Design review of the part built by this model. Coordinates are the model's own, in mm. A direction names the side the tool comes from. Coordinates: 2 decimals unless noted, no trailing zeros. Order: outer loops, then holes, each group sorted by start corner. A loop starts at its lowest first (then second) coordinate and runs counter-clockwise, first axis right, second up. Notation, with made-up numbers: M 43.5,-32 L 97.5,-32 A26 ccw 97.5,-16 Z; hole C 48.5,48.5 d2. An arc over 180 degrees is marked long. Answer as a JSON object with one key per item and string values.
from build123d import *

# Parameters (mm, degrees)
F2_W     = 2
F2_H     = 35.500896
F3_DEPTH = 89.001
F6_DEPTH = 89.001


with BuildPart() as f1:
    # F0 (on Front) → F1 (revolve)
    with BuildSketch(Plane.XZ):
        Polygon((-44.5, 45), (-44.5, 30), (44.5, 30), (44.5, 57.508134), align=None)
    revolve(axis=Axis((4.300002, 0, 0), (1, 0, 0)))

    # F2 (on face) → F3 (cut, through all)
    with BuildSketch(Plane.YZ.offset(44.5)):
        with Locations((0, -46.971067)):
            Rectangle(F2_W, F2_H)
    extrude(amount=-F3_DEPTH, mode=Mode.SUBTRACT)

    # F5 (on face) → F6 (cut, through all)
    with BuildSketch(Plane.YZ.offset(44.5)):
        Polygon((-9.3801, 23.522235), (-19.162689, 33.304824), (-33.304824, 19.162689), (-23.522235, 9.3801), align=None)
    extrude(amount=-F6_DEPTH, mode=Mode.SUBTRACT)


solid = f1.part
1) Insertion check: pin 1 Ø6 at (x, z) = (22, 20.5) entering from +Y; pin 2 Ø3 at (x, y) = (6, 46) entering from -Z; pin 3 Ø22 at (x, z) = (-1, -41) entering from -Y; pin 4 Ø10 at (y, z) = (15.5, -22) entering from +X. Each pin has a flat end and moves straight along its axis. Give the tip position at first contact, or say it passes through.
Taken from the geometry:
{"pin 1": "stops at y = 51.54", "pin 2": "stops at z = -27.12", "pin 3": "stops at y = -41.61", "pin 4": "stops at x = 44.5"}
2) Add section A-A (z = 0). State the section outline as (x, y) points.
Taken from the geometry:
{"outline": "M -44.5,-45 L 44.5,-57.51 L 44.5,-30 L -44.5,-30 Z; M -44.5,30 L 44.5,30 L 44.5,57.51 L -44.5,45 Z"}
3) To check wall thickness, follow L1, parallel to Y at x = 14, z = 0; L2, parallel to Y at x = -35, z = -17; L3, parallel to Z at x = 39, y = -14.5. State the ranges of each line that lie inside material, in increasing order.
Taken from the geometry:
{"L1": "y = -53.22 to -30, 30 to 53.22", "L2": "y = -43.1 to -24.72, 24.72 to 43.1", "L3": "z = -54.85 to -26.26, 28.64 to 54.85"}
4) Add section B-B (x = 17.5). State the section outline as (y, z) points.
Taken from the geometry:
{"outline": "M -33.3,19.16 L -19.16,33.3 L -12.93,27.07 A30 cw long 1,-29.98 L 1,-53.7 A53.71 ccw long -1,-53.7 L -1,-29.98 A30 cw -27.07,12.93 Z"}
5) Tool access review of faces 1 (the flat face through (1, 1, -41)), 2 (the cylindrical face through (0.623, -25.853, -15.219)), 3 (the flat face through (44.5, 25, -25)): name each direction out of +Z, -Z, +X, -X, +Y, -Y from which nothing blocks a thin tool from reaching the whole face with its end or side.
Taken from the geometry:
{"face 1": "-Z, +X, -X", "face 2": "+X, -X", "face 3": "+Z, -Z, +X, +Y, -Y"}
6) Mouldability with a two-part tool opening along Y and no side actions: class faces 4 (the flat face through (0.62, -30.23, 16.09)), 5 (the flat face through (0.62, -16, 30.14)), 6 (the flat face through (-44.5, 29, 9)) as released by +Y, released by -Y, zero draft, split by the parting line, or undercut.
Taken from the geometry:
{"face 4": "undercut", "face 5": "undercut", "face 6": "zero draft"}
